Geometry check sheet. Reference: the model listing, model coordinates, mm. A direction names the side the tool comes from. Round coordinates to 2 decimals unless told otherwise and drop trailing zeros. Write each loop counter-clockwise with the first axis right and the second up, starting at its lowest first coordinate (ties: lowest second). Pieces come first, ordered by that corner, then holes.
Item 1: Draft check along X on faces 3 (the face through (-110.86, -85.01, 9.41)), 4 (the face through (17.239, -109.066, 14.354)), 5 (the face through (-2, -29, 19.05)). Enter one of: pulls with the +X half, pulls with the -X half, needs draft (parallel to the pull), parting line crosses it, or undercut.
Item 2: Access from +Z, -Z, +X, -X, +Y, -Y to the whole of each face (thin tool, end or side, straight path). Record for faces 1 (the face through (-2.362, -1.811, 9.392)), 2 (the face through (17.14, -133.92, 14.35)).
Item 3: Depth check by flat-ended pin: P1, Ø7.5, axis at y = -124.5, z = 14.5, coming from the -X side; P2, Ø3, axis at y = -124.5, z = 16.5, coming from the +X side; P3, Ø4, axis at y = -93.5, z = 5.5, coming from the +X side. Enter the tip coordinate at first touch or a pass-through.
Item 4: Cross-section at A-A (z = 5.5). Enter the section's corners in (x, y).
Item 5: Scan lines: probe 1 along Y at (x, z) = (0, 9); probe 2 along Y at (x, z) = (20.5, 5.75); probe 3 along Y at (x, z) = (56.5, 16). Record each from-to range of solid material in increasing order.
from build123d import *

# Parameters (mm, degrees)
F2_R     = 139.7
F2_R_2   = 2.9765625
F3_DEPTH = 19.05
F4_SIZE  = 1.5875
F6_DEPTH = 5.55625
F8_DEPTH = 9.525


# Not quite as in the source:
# - a variable given as a bare number and used for a length is read in inches; the dataset says mm whatever the document's units were


with BuildPart() as f3:
    # F2 (on Top) → F3 (new body)
    with BuildSketch(Plane.XY):
        Circle(F2_R)
        Circle(F2_R_2, mode=Mode.SUBTRACT)
    extrude(amount=F3_DEPTH)

    # F4
    f4_edges = [f3.edges().sort_by_distance(p)[0] for p in [
        (-139.7, 0, 19.05),
        (-139.7, 0, 0),
    ]]
    chamfer(f4_edges, length=F4_SIZE)

    # F5 (on face) → F6 (cut)
    with BuildSketch(Plane.XY.offset(19.05)):
        with BuildLine():
            Line((6.35, -137.9664457622), (6.35, -114.2999987969))
            ThreePointArc((6.35, -114.2999987969), (-6.016e-07, -107.95), (-6.35, -114.3))
            Line((-6.35, -114.3), (-6.35, -137.9664457622))
            ThreePointArc((-6.35, -137.9664457622), (0, -138.1125), (6.35, -137.9664457622))
        make_face()
        with BuildLine():
            Line((6.35, -143.818885088), (6.35, -137.9664457622))
            ThreePointArc((6.35, -137.9664457622), (0, -138.1125), (-6.35, -137.9664457622))
            Line((-6.35, -137.9664457622), (-6.35, -143.818885088))
            Line((-6.35, -143.818885088), (6.35, -143.818885088))
        make_face()
    extrude(amount=-F6_DEPTH, mode=Mode.SUBTRACT)

    # F7 (on face) → F8 (cut)
    with BuildSketch(Plane.XY.offset(19.05)):
        with BuildLine():
            Line((12.7, -107.15625), (-12.7, -107.15625))
            ThreePointArc((-12.7, -107.15625), (-17.1901280605, -109.0161219395), (-19.05, -113.50625))
            Line((-19.05, -113.50625), (-19.05, -129.38125))
            ThreePointArc((-19.05, -129.38125), (-17.1901280605, -133.8713780605), (-12.7, -135.73125))
            Line((-12.7, -135.73125), (-6.35, -135.73125))
            Line((-6.35, -135.73125), (-6.35, -114.3))
            ThreePointArc((-6.35, -114.3), (-6.016e-07, -107.95), (6.35, -114.2999987969))
            Line((6.35, -114.2999987969), (6.35, -135.73125))
            Line((6.35, -135.73125), (12.7, -135.73125))
            ThreePointArc((12.7, -135.73125), (17.1901280605, -133.8713780605), (19.05, -129.38125))
            Line((19.05, -129.38125), (19.05, -113.50625))
            ThreePointArc((19.05, -113.50625), (17.1901280605, -109.0161219395), (12.7, -107.15625))
        make_face()
        with BuildLine():
            Line((-6.35, -114.3), (-6.35, -135.73125))
            Line((-6.35, -135.73125), (6.35, -135.73125))
            Line((6.35, -135.73125), (6.35, -114.2999987969))
            ThreePointArc((6.35, -114.2999987969), (-6.016e-07, -107.95), (-6.35, -114.3))
        make_face()
    extrude(amount=-F8_DEPTH, mode=Mode.SUBTRACT)


solid = f3.part
Resolved:
1. face 3: parting line crosses it
1. face 4: undercut
1. face 5: needs draft
2. face 1: +Z, -Z
2. face 2: +Z
3. P1: stops at x = -70.25
3. P2: stops at x = 66.24
3. P3: stops at x = 105.56
4. outline: circle Ø279.4 at (0, 0); hole circle Ø5.95 at (0, 0)
5. probe 1: y = -139.7 to -2.98, 2.98 to 139.7
5. probe 2: y = -138.19 to 138.19
5. probe 3: y = -127.76 to 127.76
